Work out the finished part from the listing and answer in its coordinate system (mm). A direction names the side the tool comes from. Round coordinates to 2 decimals unless told otherwise and drop trailing zeros. Order: outer loops, then holes, each group sorted by start corner. A loop starts at its lowest first (then second) coordinate and runs counter-clockwise, first axis right, second up. Notation, with made-up numbers: (18.25, 34) - (52.25, 34) arc R23 ccw to (52.25, 69) - close; hole circle Ø11 at (-37.5, 72.5). An arc over 180 degrees is marked (long way). Answer in a Markdown table with one row per item.
from build123d import *

# Parameters (mm, degrees)
SKETCH1_W           = 92.71
SKETCH1_H           = 92.71
SKETCH1_R           = 36.83
BOSS_EXTRUDE1_DEPTH = 3.175
SKETCH2_R           = 2.25
CUT_EXTRUDE1_DEPTH  = 4.175
CIRPATTERN1_COUNT   = 4
FILLET1_R           = 12.7
FILLET2_R           = 1.27


with BuildPart() as part:
    # Sketch1 → Boss-Extrude1 (new body)
    with BuildSketch(Plane(origin=(0, 0, 0), x_dir=(1, 0, 0), z_dir=(0, 1, 0))):
        Rectangle(SKETCH1_W, SKETCH1_H)
        Circle(SKETCH1_R, mode=Mode.SUBTRACT)
    extrude(amount=BOSS_EXTRUDE1_DEPTH)

    # Sketch2 → Cut-Extrude1 (cut, through all)
    with BuildSketch(Plane(origin=(0, 3.175, 0), x_dir=(1, 0, 0), z_dir=(0, 1, 0))):
        with Locations((-34.925, 34.925)):
            Circle(SKETCH2_R)
    cut_extrude1 = extrude(amount=-CUT_EXTRUDE1_DEPTH, mode=Mode.SUBTRACT)

    # CirPattern1: Cut-Extrude1 ×4 about axis
    cirpattern1_axis = Axis((0, 0, 0), (0, 1, 0))
    for i in range(1, CIRPATTERN1_COUNT):
        add(cut_extrude1.rotate(cirpattern1_axis, i * 360 / CIRPATTERN1_COUNT), mode=Mode.SUBTRACT)

    # Fillet1
    fillet1_edges = [part.edges().sort_by_distance(p)[0] for p in [
        (-46.355, 1.5875, -46.355),
        (46.355, 1.5875, -46.355),
        (46.355, 1.5875, 46.355),
        (-46.355, 1.5875, 46.355),
    ]]
    fillet(fillet1_edges, radius=FILLET1_R)

    # Sketch4 → Revolve1 (revolve)
    with BuildSketch(Plane.XY):
        Polygon((36.83, 12.7), (36.83, 3.175), (37.465, 3.175), (37.465, 10.330147737), align=None)
    revolve(axis=Axis((0, -1000, 0), (0, 1, 0)))

    # Fillet2
    fillet2_edges = [part.edges().sort_by_distance(p)[0] for p in [
        (-37.465, 3.175, 0),
        (-37.465, 10.330147737, 0),
    ]]
    fillet(fillet2_edges, radius=FILLET2_R)


solid = part.part
1) Find section A-A, the plane y = 8.75. Give the vertices of the cut face in (x, z) (3 decimals), then the cut area to 3 significant figures.
Filled in:
| item | result |
|---|---|
| outline | circle Ø74.93 at (0, 0); hole circle Ø73.66 at (0, 0) |
| area | 148 mm^2 |
2) Find the intervals of material crossed by probe 1 along Z at (x, y) = (0, 9.75) (3 decimals); probe 2 along Y at (x, z) = (-42, 23.5) (3 decimals), in increasing order. Write a range as from..to.
Filled in:
| item | result |
|---|---|
| probe 1 | z = -37.465..-36.83, 36.83..37.465 |
| probe 2 | y = 0..3.175 |
3) The mould has two halves that part along Z. Classify faces 1 (the face through (-42.73, 1.61, -42.54)), 2 (the face through (-32, 0, -21)), 3 (the face through (33.556, 1.61, -36.711)), 4 (the face through (-33.556, 1.61, 36.711)): released by +Z, released by -Z, zero draft, split by the parting line, or undercut.
Filled in:
| item | result |
|---|---|
| face 1 | released by -Z |
| face 2 | zero draft |
| face 3 | undercut |
| face 4 | undercut |
4) Find section B-B, the plane z = 40. Give the vertices of the cut face in (x, y) (3 decimals).
Filled in:
| item | result |
|---|---|
| outline | (-44.656, 0) - (44.656, 0) - (44.656, 3.175) - (-44.656, 3.175) - close |
5) Which of the six approach directions +Z, -Z, +X, -X, +Y, -Y give full straight-line access (tool end or side, diameter ignored) to faces 5 (the face through (35.735, 7.344, -11.253)), 6 (the face through (0, 2, 46.355))?
Filled in:
| item | result |
|---|---|
| face 5 | +Y |
| face 6 | +Z, +X, -X, +Y, -Y |
6) Each of these flat-tipped pins is pushed along its axis until it touches: pin 1 (6 mm diameter, centred on y = 10, z = -19.5, fed in from -X); pin 2 (7 mm diameter, centred on x = -34.925, z = -34.925, fed in from +Y) (3 decimals); pin 3 (1 mm diameter, centred on y = 10, z = -14.5, fed in from -X). Where does it stop, or does it pass through?
Filled in:
| item | result |
|---|---|
| pin 1 | stops at x = -33.64 |
| pin 2 | stops at y = 3.175 |
| pin 3 | stops at x = -34.75 |
